Check sheet for the modelled part. Datum: model origin and axes. Units: mm. A direction names the side the tool comes from. Round coordinates to 2 decimals unless told otherwise and drop trailing zeros. Write each loop counter-clockwise with the first axis right and the second up, starting at its lowest first coordinate (ties: lowest second). Pieces come first, ordered by that corner, then holes. Notation, with made-up numbers: (88, 36.5) - (97, 36.5) arc R24 cw to (97, 62.5) - close; hole circle Ø4 at (-5.5, 3.25). An arc over 180 degrees is marked (long way). Answer as a JSON object with one key per item and string values. Group by question number.
Item 1: Thickness scan on line 1 (Y direction, x = 11, z = -1.5); line 2 (X direction, y = 259, z = -2.25); line 3 (Z direction, x = 23.5, y = 32). Record the ranges inside material, lowest first.
Item 2: Release check for a two-part mould opening along Z. For faces 4 (the flat face through (13, 176, -1.588)), 5 (the flat face through (0.4, 75.019, -13.3)), 6 (the flat face through (13, 138, 0)) record: pulls with the +Z half, pulls with the -Z half, needs draft (parallel to the pull), parting line crosses it, or undercut.
Item 3: Sectioned sample at C-C on y = 100. Record the boundary of the cut face in (x, z), plus the area to 3 significant figures.
Item 4: Sectioned sample at B-B on x = 20.5. Record the boundary of the cut face in (y, z), plus the area to 3 significant figures.
Item 5: Set-up check for faces 1 (the flat face through (7, 279.4, -1)), 2 (the flat face through (13, 24, -1.588)), 3 (the flat face through (13, 62, -1.084)): record each of +Z, -Z, +X, -X, +Y, -Y from which the full face is reachable in a straight line by a thin tool's end or side.
Item 6: Sectioned sample at D-D on y = 71.5. Record the boundary of the cut face in (x, z).
Item 7: Sectioned sample at A-A on z = -18. Record the boundary of the cut face in (x, y).
Item 8: Gauge pin test, flat ends, axial feed: P1, Ø12, axis at x = 15.5, z = -9.5, coming from the -Y side; P2, Ø12, axis at x = 17.5, y = 184.5, coming from the -Z side; P3, Ø12.5, axis at x = 10.5, y = 58.5, coming from the -Z side; P4, Ø6, axis at x = 3, y = 234, coming from the -Z side. Record the tip position at first contact, or that the pin passes through.
```python
from build123d import *

# Parameters (mm, degrees)
BOSS_EXTRUDE1_DEPTH = 279.4
SKETCH4_W           = 24.315928
SKETCH4_H           = 25.4
CUT_EXTRUDE1_DEPTH  = 26.4


with BuildPart() as part:
    # Sketch1 → Boss-Extrude1 (new body)
    with BuildSketch(Plane(origin=(0, 0, 0), x_dir=(1, 0, 0), z_dir=(0, 1, 0))):
        Polygon((0, 0), (0, 25.4), (1.5875, 25.4), (1.5875, 1.5875), (25.4, 1.5875), (25.4, 0), align=None)
    extrude(amount=BOSS_EXTRUDE1_DEPTH)

    # Sketch4 → Cut-Extrude1 (cut, through all)
    with BuildSketch(Plane.ZY):
        with Locations((-13.242036, 62.3189)):
            Rectangle(SKETCH4_W, SKETCH4_H)
    extrude(amount=-CUT_EXTRUDE1_DEPTH, mode=Mode.SUBTRACT)


solid = part.part
```
Completed:
{
 "1": {"line 1": "0 to 49.62, 75.02 to 279.4", "line 2": "0 to 1.59", "line 3": "-1.59 to 0"},
 "2": {"face 4": "pulls with the -Z half", "face 5": "needs draft", "face 6": "pulls with the +Z half"},
 "3": {"outline": "(0, -25.4) - (1.59, -25.4) - (1.59, -1.59) - (25.4, -1.59) - (25.4, 0) - (0, 0) - close", "area": "78.1 mm²"},
 "4": {"outline": "(0, -1.59) - (49.62, -1.59) - (49.62, -1.08) - (75.02, -1.08) - (75.02, -1.59) - (279.4, -1.59) - (279.4, 0) - (0, 0) - close", "area": "431 mm²"},
 "5": {"face 1": "+Z, -Z, +X, -X, +Y", "face 2": "-Z, +X, +Y, -Y", "face 3": "-Z, +X, -X"},
 "6": {"outline": "(0, -1.08) - (25.4, -1.08) - (25.4, 0) - (0, 0) - close"},
 "7": {"outline": "(0, 0) - (1.59, 0) - (1.59, 49.62) - (0, 49.62) - close; (0, 75.02) - (1.59, 75.02) - (1.59, 279.4) - (0, 279.4) - close"},
 "8": {"P1": "through", "P2": "z = -1.59", "P3": "z = -1.08", "P4": "z = -25.4"}
}
